The model under review builds one solid part; all positions refer to its coordinate system, in mm. A direction names the side the tool comes from. Give positions to 0.01 mm unless a question says otherwise; leave off trailing zeros. Loops run counter-clockwise (first coordinate to the right, second up) from the corner with the lowest first, then second, coordinate; pieces in that order, holes last. Notation, with made-up numbers: M 50.5,11.5 L 57.5,11.5 A21 ccw 57.5,31.5 Z; hole C 48.5,27 d4. An arc over 180 degrees is marked long. One line per item, written item: value. Start each with the question number.
Q1. For pin 1 (20 mm diameter, centred on y = 55.5, z = 22, fed in from +X); pin 2 (1.4 mm diameter, centred on x = -12.5, z = -1, fed in from -Y); pin 3 (4 mm diameter, centred on x = -10.9, y = 5.74, fed in from +Z), all flat-tipped, find the tip position at first contact; note any pin that passes through.
Q2. We need section C-C on z = 45.5. Write out the cut boundary in (x, y), plus the area to 3 significant figures.
Q3. We need section A-A on x = -7. Write out the cut boundary in (y, z), plus the area to 3 significant figures.
Q4. We need section D-D on z = 7. Write out the cut boundary in (x, y).
Q5. To check wall thickness, follow line 1 along Y through (x, z) = (-10.9, -1); line 2 along X through (y, z) = (-0.25, 40); line 3 along Y through (x, z) = (-14, 33). State the ranges of each line that lie inside material, in increasing order. Write a range as from..to.
Q6. For faces 4 (the face through (-9, 58, -1.237)), 5 (the face through (-8, 0, 25)), list the 3-axis set-ups (+Z, -Z, +X, -X, +Y, -Y) from which the entire face can be reached by the end or side of a thin tool; tool diameter is ignored.
Q7. Mouldability with a two-part tool opening along Z and no side actions: class faces 1 (the face through (-9, 58, -0.737)), 2 (the face through (-15.99, 35.64, 18.38)), 3 (the face through (-15.737, 46, 15)) as released by +Z, released by -Z, zero draft, split by the parting line, or undercut.
Q8. We need section B-B on y = 56. Write out the cut boundary in (x, z), plus the area to 3 significant figures.
```python
from build123d import *

# Parameters (mm, degrees)
SKETCH2_W          = 15
SKETCH2_H          = 50
BASE_FLANGE1_DEPTH = 0.5
EDGE_FLANGE1_DEPTH = 50
CUT_EXTRUDE1_DEPTH = 10
EDGE_FLANGE2_DEPTH = 115.2634
CUT_EXTRUDE2_DEPTH = 10
SKETCH13_R         = 1.5
CUT_EXTRUDE3_DEPTH = 10
SKETCH14_R         = 1.5
CUT_EXTRUDE4_DEPTH = 10
SKETCH15_R         = 2
CUT_EXTRUDE5_DEPTH = 12
SKETCH16_R         = 2
CUT_EXTRUDE6_DEPTH = 12


# Sheet-metal steps are written as plain solids
with BuildPart() as part:
    # Sketch2 → Base-Flange1 (new body)
    with BuildSketch(Plane(origin=(0, 0, 0), x_dir=(1, 0, 0), z_dir=(0, 1, 0))):
        with Locations((-7.5, -25)):
            Rectangle(SKETCH2_W, SKETCH2_H)
    extrude(amount=-BASE_FLANGE1_DEPTH)

    # Edge-Flange1 section (across the edge) → Edge-Flange1 (add)
    with BuildSketch(Plane(origin=(-15.7366, 0, 0), x_dir=(1, 0, 0), z_dir=(0, 0, 1))):
        with BuildLine():
            Line((-0.5, 0.7366), (-0.5, 116))
            Line((-0.5, 116), (0, 116))
            Line((0, 116), (0, 0.7366))
            ThreePointArc((0, 0.7366), (0.215745145, 0.215745145), (0.7366, 0))
            Line((0.7366, 0), (0.7366, -0.5))
            ThreePointArc((0.7366, -0.5), (-0.137808246, -0.137808246), (-0.5, 0.7366))
        make_face()
    extrude(amount=EDGE_FLANGE1_DEPTH)

    # Sketch8 → Cut-Extrude1 (cut)
    with BuildSketch(Plane.ZY.offset(16.2366)):
        Polygon((40, 0.7366), (0, 116), (50, 116), (50, 0.7366), align=None)
    extrude(amount=-CUT_EXTRUDE1_DEPTH, mode=Mode.SUBTRACT)

    # Edge-Flange2 section (across the edge) → Edge-Flange2 (add)
    with BuildSketch(Plane(origin=(-15.7366, 0.7366, -0.7366), x_dir=(0, 0, 1), z_dir=(0, 1, 0))):
        with BuildLine():
            Line((-0.5, 0.7366), (-0.5, 12))
            Line((-0.5, 12), (0, 12))
            Line((0, 12), (0, 0.7366))
            ThreePointArc((0, 0.7366), (0.215745145, 0.215745145), (0.7366, 0))
            Line((0.7366, 0), (0.7366, -0.5))
            ThreePointArc((0.7366, -0.5), (-0.137808246, -0.137808246), (-0.5, 0.7366))
        make_face()
    extrude(amount=EDGE_FLANGE2_DEPTH)

    # Sketch12 → Cut-Extrude2 (cut)
    with BuildSketch(Plane.ZY.offset(16.2366)):
        Polygon((10, 59.851091606), (27, 10.7366), (10, 10.7366), align=None)
    extrude(amount=-CUT_EXTRUDE2_DEPTH, mode=Mode.SUBTRACT)

    # Sketch13 → Cut-Extrude3 (cut)
    with BuildSketch(Plane(origin=(0, 0, -1.2366), x_dir=(-1, 0, 0), z_dir=(0, 0, -1))):
        with Locations((10.9, 5.7366)):
            Circle(SKETCH13_R)
    extrude(amount=-CUT_EXTRUDE3_DEPTH, mode=Mode.SUBTRACT)

    # Sketch14 → Cut-Extrude4 (cut)
    with BuildSketch(Plane.XY.offset(-0.7366)):
        with Locations((-10.9, 112.5366)):
            Circle(SKETCH14_R)
    extrude(amount=-CUT_EXTRUDE4_DEPTH, mode=Mode.SUBTRACT)

    # Sketch15 → Cut-Extrude5 (cut)
    with BuildSketch(Plane(origin=(0, 0, 0), x_dir=(1, 0, 0), z_dir=(0, 1, 0))):
        with Locations(Location((-7, -40, 0), (0, 0, 270))):
            Circle(SKETCH15_R)
    extrude(amount=-CUT_EXTRUDE5_DEPTH, mode=Mode.SUBTRACT)

    # Sketch16 → Cut-Extrude6 (cut)
    with BuildSketch(Plane(origin=(0, 0, 0), x_dir=(1, 0, 0), z_dir=(0, 1, 0))):
        with Locations(Location((-7, -7, 0), (0, 0, 270))):
            Circle(SKETCH16_R)
    extrude(amount=-CUT_EXTRUDE6_DEPTH, mode=Mode.SUBTRACT)


solid = part.part
```
Solved:
1. pin 1: x = -15.74
1. pin 2: y = 0.74
1. pin 3: z = -0.74
2. outline: M -16.24,0.74 A1.24 ccw -15,-0.5 L 0,-0.5 L 0,0 L -15,0 A0.74 cw -15.74,0.74 Z
2. area: 8.27 mm2
3. outline: M -0.5,0 L 0,0 L 0,5 L -0.5,5 Z; M -0.5,9 L 0,9 L 0,38 L -0.5,38 Z; M -0.5,42 L 0,42 L 0,50 L -0.5,50 Z; M 0.74,-1.24 L 116,-1.24 L 116,-0.74 L 0.74,-0.74 Z
3. area: 78.6 mm2
4. outline: M -16.24,0.74 A1.24 ccw -15,-0.5 L -9,-0.5 L -9,0 L -15,0 A0.74 cw -15.74,0.74 L -15.74,95.83 L -16.24,95.83 Z; M -5,-0.5 L 0,-0.5 L 0,0 L -5,0 Z
5. line 1: 0.74..4.24, 7.24..111.04, 114.04..116
5. line 2: -15.75..-9, -5..0
5. line 3: -0.5..0
6. face 4: -Z, +X, -X, +Y, -Y
6. face 5: +Z, -Z, +X, +Y
7. face 1: released by +Z
7. face 2: undercut
7. face 3: zero draft
8. outline: M -16.24,0 A1.24 ccw -15,-1.24 L -3.74,-1.24 L -3.74,-0.74 L -15,-0.74 A0.74 cw -15.74,0 L -15.74,10 L -16.24,10 Z; M -16.24,11.33 L -15.74,11.33 L -15.74,20.82 L -16.24,20.82 Z
8. area: 16.2 mm2
